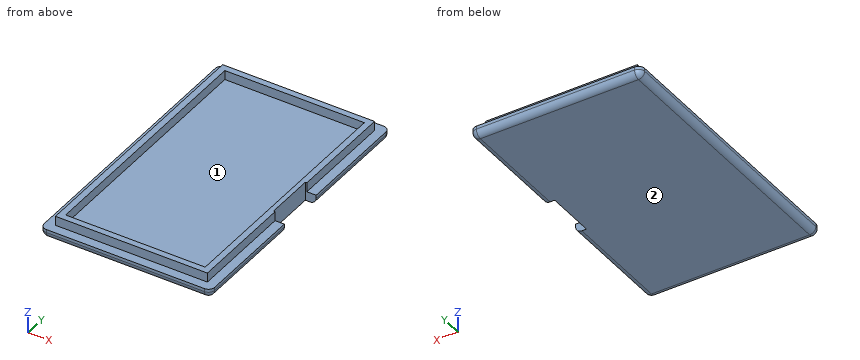
Autodesk Inventor part; units mm, degrees
ref_plane "YZ Plane" through (0, 0, 0) normal (1, 0, 0) x (0, 1, 0)
ref_plane "XZ Plane" through (0, 0, 0) normal (0, 1, 0) x (-1, 0, 0)
ref_plane "XY Plane" through (0, 0, 0) normal (0, 0, 1) x (1, 0, 0)
sketch "Náčrt1" plane through (0, 0, 0) normal (0, 0, 1) x (1, 0, 0)
  line L0 (0, 63) -> (0, -63)
  line L1 (-38.5, 0) -> (38.5, 0)
  line L2 (27.5, -45) -> (-27.5, -45)
  line L3 (-27.5, -45) -> (-27.5, 45)
  line L4 (-27.5, 45) -> (27.5, 45)
  line L5 (27.5, 45) -> (27.5, -45)
  point P0 (0, 0)
  dimension "d0" = 55
  dimension "d1" = 90
extrude "Vysunutí1" add sketch "Náčrt1" along normal blind 3
sketch "Náčrt2" plane through (0, 0, 3) normal (0, 0, 1) x (1, 0, 0)
  line L0 (27.5, 45) -> (-27.5, 45)
  line L1 (-27.5, 45) -> (-27.5, -45)
  line L2 (-27.5, -45) -> (27.5, -45)
  line L3 (27.5, -45) -> (27.5, 45)
  line L4 (-27.5, 45) -> (-27.5, -45)
  line L5 (0, 63) -> (0, -63)
  line L6 (-38.5, 0) -> (38.5, 0)
  line L7 (24.5, -42) -> (-24.5, -42)
  line L8 (-24.5, -42) -> (-24.5, 42)
  line L9 (-24.5, 42) -> (24.5, 42)
  line L10 (24.5, 42) -> (24.5, -42)
  line L11 (-22.5, 40) -> (-22.5, -40)
  line L12 (-22.5, -40) -> (22.5, -40)
  line L13 (22.5, -40) -> (22.5, 40)
  line L14 (22.5, 40) -> (-22.5, 40)
  line L15 (-22.5, 0) -> (-24.5, 0)
  line L16 (-24.5, 0) -> (-24.5, -42)
  line L17 (-24.5, -42) -> (-22.5, -42)
  line L18 (-22.5, -42) -> (-22.5, 0)
  line L19 (22.5, 0) -> (24.5, 0)
  line L20 (24.5, 0) -> (24.5, -42)
  line L21 (24.5, -42) -> (22.5, -42)
  line L22 (22.5, -42) -> (22.5, 0)
  line L23 (24.5, -42) -> (-22.5, -42)
  line L24 (-22.5, -42) -> (-22.5, -40)
  line L25 (-22.5, -40) -> (24.5, -40)
  line L26 (24.5, -40) -> (24.5, -42)
  line L27 (-24.5, -42) -> (-22.5, -42)
  line L28 (-22.5, -42) -> (-22.5, -40)
  line L29 (-22.5, -40) -> (-24.5, -40)
  line L30 (-24.5, -40) -> (-24.5, -42)
  point P0 (0, 0)
  point P1 (24.5, 0)
  dimension "d8" = 49
  dimension "d9" = 84
  dimension "d10" = 2
extrude "Vysunutí2" add sketch "Náčrt2" along normal blind 3 contours L9 L10 L6 L13 L14 L5 | L5 L14 L11 L6 L8 L9 | L10 L25 L13 L6 | L10 L7 L22 L25 | L6 L11 L29 L8 | L7 L18 L12 L5 | L5 L12 L22 L7 | L29 L18 L7 L8
sketch "Náčrt3" plane through (0, 0, 0) normal (0, 0, -1) x (-1, 0, 0)
  line L0 (-27.5, 45) -> (27.5, 45)
  line L1 (-27.5, -45) -> (-27.5, 45)
  line L2 (27.5, -45) -> (-27.5, -45)
  line L3 (27.5, 45) -> (27.5, -45)
  line L4 (-27.5, -8) -> (-24, -8)
  line L5 (-24, -8) -> (-24, 8)
  line L6 (-24, 8) -> (-27.5, 8)
  line L7 (-27.5, 8) -> (-27.5, -8)
  line L8 (0, -63) -> (0, 63)
  line L9 (-38.5, 0) -> (38.5, 0)
  point P0 (0, 0)
  point P1 (-27.5, 8)
  dimension "d13" = 3.5
  dimension "d14" = 16
extrude "Vysunutí3" cut sketch "Náčrt3" against normal through all contours L6 L5 L9 L1 | L9 L5 L4 L1
fillet "Zaoblení1" radius 2 9 edges at (27.5, 26.5, 0) (0, 45, 0) (27.5, 45, 1.5) (-27.5, 45, 1.5) (-27.5, 0, 0) (27.5, -26.5, 0) (0, -45, 0) (27.5, -45, 1.5) (-27.5, -45, 1.5)
properties part number "adapter_box_lid_3D tisk"
Here's how the part is built. I have some questions about the finished solid (model axes, mm). Face numbers are marked on the shaded views. Round coordinates to 2 decimals unless told otherwise and drop trailing zeros. Order: outer loops, then holes, each group sorted by start corner. A loop starts at its lowest first (then second) coordinate and runs counter-clockwise, first axis right, second up. Notation, with made-up numbers: (0.5, 70.5) -> (33.5, 70.5) arc R26 cw to (33.5, 91.5) -> close; hole circle Ø10 at (78.5, 45.25). An arc over 180 degrees is marked (long way). Use a Markdown table: item, result. Add a question column.
(1) Suppose I cut it at D-D, the plane y = -6. Please give me the cut outline in (x, z), and give its area (3 significant figures).
(2) If we mould it in two halves opening along X, with no side actions, what happens to the marked faces 1 and 2? For each: released by +X, released by -X, zero draft, split by the parting line, or undercut.
(3) Suppose I cut it at C-C, the plane x = 10. Please give me the cut outline in (y, z), and give its area (3 significant figures).
(4) Suppose I cut it at A-A, the plane z = 4.65. Please give me the cut outline in (x, y), and give its area (3 significant figures).
(5) I need wall thicknesses on line 1 along X through (y, z) = (39, 3.3); line 2 along Y through (x, z) = (3.5, 5.15); line 3 along Z through (x, y) = (25, 34.5). Which ranges of each line are inside material? Lowest first, please.
(6) For pin 1 Ø22.5 at (x, y) = (-1, 18) entering from +Z; pin 2 Ø1.5 at (x, z) = (-3.5, 5) entering from -Y; pin 3 Ø0.9 at (y, z) = (-23, 4.5) entering from +X, each with a flat end and sliding along its axis, tell me the tip position at first contact or that it passes through.
(7) Suppose I cut it at B-B, the plane y = 19.5. Please give me the cut outline in (x, z), and give its area (3 significant figures).
Verdict:
| question | item | result |
|---|---|---|
| 1 | outline | (-27.5, 2) arc R2 ccw to (-25.5, 0) -> (24, 0) -> (24, 6) -> (22.5, 6) -> (22.5, 3) -> (-22.5, 3) -> (-22.5, 6) -> (-24.5, 6) -> (-24.5, 3) -> (-27.5, 3) -> close |
| 1 | area | 164 mm2 |
| 2 | face 1 | undercut |
| 2 | face 2 | zero draft |
| 3 | outline | (-45, 2) arc R2 ccw to (-43, 0) -> (43, 0) arc R2 ccw to (45, 2) -> (45, 3) -> (42, 3) -> (42, 6) -> (40, 6) -> (40, 3) -> (-40, 3) -> (-40, 6) -> (-42, 6) -> (-42, 3) -> (-45, 3) -> close |
| 3 | area | 280 mm2 |
| 4 | outline | (-24.5, -42) -> (24.5, -42) -> (24.5, -8) -> (24, -8) -> (24, 8) -> (24.5, 8) -> (24.5, 42) -> (-24.5, 42) -> close; hole (-22.5, -40) -> (22.5, -40) -> (22.5, 40) -> (-22.5, 40) -> close |
| 4 | area | 508 mm2 |
| 5 | line 1 | -24.5 to -22.5, 22.5 to 24.5 |
| 5 | line 2 | -42 to -40, 40 to 42 |
| 5 | line 3 | 0 to 3 |
| 6 | pin 1 | z = 3 |
| 6 | pin 2 | y = -42 |
| 6 | pin 3 | x = 24.5 |
| 7 | outline | (-27.5, 2) arc R2 ccw to (-25.5, 0) -> (25.5, 0) arc R2 ccw to (27.5, 2) -> (27.5, 3) -> (24.5, 3) -> (24.5, 6) -> (22.5, 6) -> (22.5, 3) -> (-22.5, 3) -> (-22.5, 6) -> (-24.5, 6) -> (-24.5, 3) -> (-27.5, 3) -> close |
| 7 | area | 175 mm2 |
